from build123d import *

# Parameters (mm, degrees)
EXTRUDE_1_DEPTH     = 15
SKETCH_2_R          = 1.5
CUT_EXTRUDE_1_DEPTH = 3
SKETCH_3_R          = 1.5
CUT_EXTRUDE_2_DEPTH = 3
EXTRUDE_2_DEPTH     = 2
EXTRUDE_3_DEPTH     = 2
SKETCH_6_R          = 1.4
CUT_EXTRUDE_3_DEPTH = 27.645825189
FILLET_1_R          = 3


with BuildPart() as part:
    # 草图1 → 凸台-拉伸1 (new body)
    with BuildSketch(Plane.XY):
        Polygon((0, -14), (0, 0), (17, 0), (17, 3), (-3, 3), (-3, -14), align=None)
    extrude(amount=EXTRUDE_1_DEPTH)

    # 草图2 → 切除-拉伸1 (cut)
    with BuildSketch(Plane(origin=(0, 0, 0), x_dir=(0, 0, -1), z_dir=(1, 0, 0))):
        with Locations(Location((-7.5, -6, 0), (0, 0, 90))):
            Circle(SKETCH_2_R)
    extrude(amount=-CUT_EXTRUDE_1_DEPTH, mode=Mode.SUBTRACT)

    # 草图3 → 切除-拉伸2 (cut)
    with BuildSketch(Plane.XZ):
        with Locations(Location((13, 7.5, 0), (0, 0, 270))):
            Circle(SKETCH_3_R)
        with Locations(Location((5, 7.5, 0), (0, 0, 270))):
            Circle(SKETCH_3_R)
    extrude(amount=-CUT_EXTRUDE_2_DEPTH, mode=Mode.SUBTRACT)

    # 草图4 → 凸台-拉伸2 (add)
    with BuildSketch(Plane.XY.offset(15)):
        Polygon((0, 0), (0, -10), (13, 0), align=None)
    extrude(amount=-EXTRUDE_2_DEPTH)

    # 草图5 → 凸台-拉伸3 (add)
    with BuildSketch(Plane(origin=(0, 0, 0), x_dir=(-1, 0, 0), z_dir=(0, 0, -1))):
        Polygon((0, 0), (-13, 0), (0, -10), align=None)
    extrude(amount=-EXTRUDE_3_DEPTH)

    # 草图6 → 切除-拉伸3 (cut, through all)
    with BuildSketch(Plane(origin=(0, 0, 0), x_dir=(-1, 0, 0), z_dir=(0, 0, -1))):
        with Locations((-3, -2)):
            Circle(SKETCH_6_R)
    extrude(amount=-CUT_EXTRUDE_3_DEPTH, mode=Mode.SUBTRACT)

    # 圆角1
    fillet_1_edges = [part.edges().sort_by_distance(p)[0] for p in [
        (0, 0, 7.5),
    ]]
    fillet(fillet_1_edges, radius=FILLET_1_R)


solid = part.part
Could you check a few things on this model? Use its own coordinates, in mm. A direction names the side the tool comes from. Give positions to 0.01 mm unless a question says otherwise; leave off trailing zeros. Write each loop counter-clockwise with the first axis right and the second up, starting at its lowest first coordinate (ties: lowest second). Pieces come first, ordered by that corner, then holes. Notation, with made-up numbers: (39.5, -18) -> (88.5, -18) arc R25 cw to (88.5, 21) -> close; hole circle Ø9 at (20.25, 82.5). An arc over 180 degrees is marked (long way). Write each question's results on one line, items separated by ' | '. Start each with the question number.
Q1. I'm going to push flat-ended pins straight in: pin 1 Ø1.8 at (x, z) = (5, 7.5) entering from +Y; pin 2 Ø2 at (x, z) = (7.5, 13) entering from -Y; pin 3 Ø1 at (y, z) = (-2, 3.5) entering from +X; pin 4 Ø3.5 at (y, z) = (-7, 6) entering from +X. Where does each tip first touch, or does it pass through?
Q2. Which directions (+Z, -Z, +X, -X, +Y, -Y) give clear straight access to the entire face, cutting with the end or side of a thin tool? Please do faces 5 (the face through (5, -4, 13)), 6 (the face through (6.41, -5.07, 14.01)).
Q3. We'd pull the mould along X, two halves only. Please class faces 1 (the face through (5, -2, 15)), 2 (the face through (2.25, -0.82, 0.99)), 3 (the face through (5, 1, 9)), 4 (the face through (6.59, -4.93, 0.99)): +X half, -X half, draft (parallel to the pull), parting line (faces both ways), or undercut.
Q4. Suppose I cut it at A-A, the plane y = -6. List the corners of the cut face in (x, z) for me.
Q5. Suppose I cut it at C-C, the plane z = 12.25. List the corners of the cut face in (x, y) for me, and give its area (3 significant figures).
Q6. I need wall thicknesses on probe 1 along Z at (x, y) = (3.5, -4.25); probe 2 along X at (y, z) = (-8.5, 9.5); probe 3 along Y at (x, z) = (9.5, 5). Which ranges of each line are inside material? Lowest first, please.
Q7. Suppose I cut it at B-B, the plane z = 7.5. List the corners of the cut face in (x, y) for me, and give its area (3 significant figures).
Q8. Suppose I cut it at D-D, the plane x = 3.25. List the corners of the cut face in (y, z) for me.
Outcome:
1) pin 1: through | pin 2: y = -5 | pin 3: x = 0.4 | pin 4: x = 0
2) face 5: +X, -Y | face 6: +Z, -Z, +X, -Y
3) face 1: draft | face 2: undercut | face 3: undercut | face 4: +X half
4) outline: (-3, 0) -> (5.2, 0) -> (5.2, 2) -> (0, 2) -> (0, 6) -> (-3, 6) -> close; (-3, 9) -> (0, 9) -> (0, 13) -> (5.2, 13) -> (5.2, 15) -> (-3, 15) -> close
5) outline: (-3, -14) -> (0, -14) -> (0, -3) arc R3 cw to (3, 0) -> (17, 0) -> (17, 3) -> (-3, 3) -> close | area: 104 mm2
6) probe 1: 0 to 2, 13 to 15 | probe 2: -3 to 0 | probe 3: 0 to 3
7) outline: (-3, -14) -> (0, -14) -> (0, -7.5) -> (-3, -7.5) -> close; (-3, -4.5) -> (0, -4.5) -> (0, -3) arc R3 cw to (3, 0) -> (3.5, 0) -> (3.5, 3) -> (-3, 3) -> close; (6.5, 0) -> (11.5, 0) -> (11.5, 3) -> (6.5, 3) -> close; (14.5, 0) -> (17, 0) -> (17, 3) -> (14.5, 3) -> close | area: 76.9 mm2
8) outline: (-7.5, 0) -> (-3.38, 0) -> (-3.38, 2) -> (-7.5, 2) -> close; (-7.5, 13) -> (-3.38, 13) -> (-3.38, 15) -> (-7.5, 15) -> close; (-0.62, 0) -> (3, 0) -> (3, 15) -> (-0.62, 15) -> (-0.62, 13) -> (0, 13) -> (0, 2) -> (-0.62, 2) -> close
